Autodesk Inventor part; units mm, degrees
ref_plane "YZ Plane" through (0, 0, 0) normal (1, 0, 0) x (0, 1, 0)
ref_plane "XZ Plane" through (0, 0, 0) normal (0, 1, 0) x (-1, 0, 0)
ref_plane "XY Plane" through (0, 0, 0) normal (0, 0, 1) x (1, 0, 0)
sketch "Sketch1" plane through (0, 0, 0) normal (0, 0, 1) x (1, 0, 0)
  circle A0 centre (0, 0) radius 8
  dimension "d0" = 16
extrude "Extrusion1" add sketch "Sketch1" against normal blind 18.5
sketch "Sketch2" plane through (0, 0, 0) normal (0, 0, 1) x (1, 0, 0)
  line L0 (-9, 9) -> (9, 9)
  line L1 (9, 9) -> (9, -9)
  line L2 (9, -9) -> (-9, -9)
  line L3 (-9, -9) -> (-9, 9)
  point P0 (0, 0)
  dimension "d3" = 18
  dimension "d4" = 18
  dimension "d5" = 9
  dimension "d6" = 9
extrude "Extrusion2" add sketch "Sketch2" along normal blind 2
sketch "Sketch3" plane through (0, 0, 2) normal (0, 0, 1) x (1, 0, 0)
  circle A0 centre (0, 0) radius 6.5
  dimension "d9" = 13
extrude "Extrusion3" add sketch "Sketch3" along normal blind 4.3
fillet "Fillet1" radius 2 4 edges at (9, 9, 1) (-9, 9, 1) (9, -9, 1) (-9, -9, 1)
properties part number "Button"
Verification items for the finished model (mm, model axes). A direction names the side the tool comes from. Round coordinates to 2 decimals unless told otherwise and drop trailing zeros. Loops run counter-clockwise (first coordinate to the right, second up) from the corner with the lowest first, then second, coordinate; pieces in that order, holes last. Notation, with made-up numbers: (-36, 5.25) - (-9, 5.25) arc R27 cw to (-9, 23.25) - close; hole circle Ø9 at (48, 72). An arc over 180 degrees is marked (long way). Use a Markdown table: item, result. Add a question column.
1. Gauge pin test, flat ends, axial feed: pin 1 (1.5 mm diameter, centred on x = 0, z = -11, fed in from +Y); pin 2 (5 mm diameter, centred on x = -6.5, z = -9, fed in from -Y); pin 3 (8 mm diameter, centred on x = -3, z = -16, fed in from -Y). Record the tip position at first contact, or that the pin passes through.
2. Section check A-A, the plane x = 0. Record the boundary of the cut face in (y, z).
3. Access from +Z, -Z, +X, -X, +Y, -Y to the whole of each face (thin tool, end or side, straight path). Record for faces 1 (the face through (-6, 4, 2)), 2 (the face through (-1.73, -7.81, -9.12)), 3 (the face through (0, 0, 6.3)).
4. Thickness scan on probe 1 along Z at (x, y) = (-5.75, 5.5); probe 2 along Z at (x, y) = (7.25, 4); probe 3 along Y at (x, z) = (3, -9.25). Record the ranges inside material, lowest first. Write a range as [from, to].
5. Section check D-D, the plane z = -11. Record the boundary of the cut face in (x, y), plus the area to 3 significant figures.
6. Section check C-C, the plane z = 4. Record the boundary of the cut face in (x, y).
Checks:
| question | item | result |
|---|---|---|
| 1 | pin 1 | stops at y = 8 |
| 1 | pin 2 | stops at y = -6.93 |
| 1 | pin 3 | stops at y = -8 |
| 2 | outline | (-9, 0) - (-8, 0) - (-8, -18.5) - (8, -18.5) - (8, 0) - (9, 0) - (9, 2) - (6.5, 2) - (6.5, 6.3) - (-6.5, 6.3) - (-6.5, 2) - (-9, 2) - close |
| 3 | face 1 | +Z |
| 3 | face 2 | -Z |
| 3 | face 3 | +Z, +X, -X, +Y, -Y |
| 4 | probe 1 | z = [-18.5, 2] |
| 4 | probe 2 | z = [0, 2] |
| 4 | probe 3 | y = [-7.42, 7.42] |
| 5 | outline | circle Ø16 at (0, 0) |
| 5 | area | 201 mm^2 |
| 6 | outline | circle Ø13 at (0, 0) |
